```python
from build123d import *

# Parameters (mm, degrees)
F0_W     = 14.2082790844
F0_H     = 68.7680318952
F0_W_2   = 16.8297942728
F1_DEPTH = 25.4
F2_R     = 10.9503541364
F3_DEPTH = 9.4174239784
F5_W     = 35.7930406462
F5_H     = 20.7620039582
F6_DEPTH = 71.0562486202


with BuildPart() as f1:
    # F0 (on Top) → F1 (new body)
    with BuildSketch(Plane.XY):
        Polygon((3.0717435293, 45.1143532991), (19.8212694377, 45.1143532991), (19.8212694377, 99.9910533428), (-35.7833579183, 99.9910533428), (-35.7833579183, 72.552703321), (-11.1365355551, 72.552703321), (-11.1365355551, 45.1143532991), align=None)
        with Locations((-4.0323960129, 10.7303373516)):
            Rectangle(F0_W, F0_H)
        with Locations((-19.5514326915, 10.7303373516)):
            Rectangle(F0_W_2, F0_H)
        Polygon((-27.9663298279, 45.1143532991), (-11.1365355551, 45.1143532991), (-11.1365355551, 72.552703321), (-35.7833579183, 72.552703321), (-35.7833579183, 45.1143532991), align=None)
        Polygon((-27.9663298279, -23.653678596), (-27.9663298279, 45.1143532991), (-35.7833579183, 45.1143532991), (-35.7833579183, 0), (-35.7833579183, -47.0235422254), (-11.1365355551, -47.0235422254), (-11.1365355551, -23.653678596), align=None)
    extrude(amount=F1_DEPTH)

    # F2 (on face) → F3 (join)
    with BuildSketch(Plane.XY.offset(25.4)):
        with Locations((-13.6862043291, 22.343069315)):
            Circle(F2_R)
    extrude(amount=F3_DEPTH)

    # F5 (on face) → F6 (join)
    with BuildSketch(Plane.XY.offset(25.4)):
        with Locations((-6.4500138396, 73.0364732444)):
            Rectangle(F5_W, F5_H)
    extrude(amount=F6_DEPTH)


solid = f1.part
```
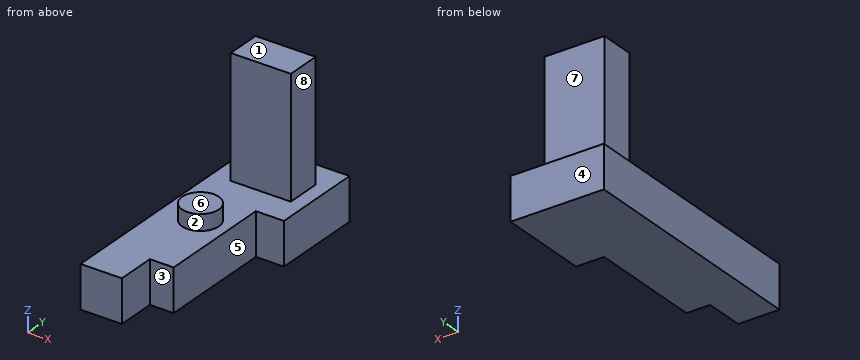
CAD build for the part. Positions are in the model's coordinates, mm. Face numbers are marked on the shaded views. A direction names the side the tool comes from. Give positions to 0.01 mm unless a question says otherwise; leave off trailing zeros. Loops run counter-clockwise (first coordinate to the right, second up) from the corner with the lowest first, then second, coordinate; pieces in that order, holes last. Notation, with made-up numbers: M 55.25,40.25 L 84.25,40.25 A15 cw 84.25,59.25 Z; hole C 56.5,-39.75 d11. An arc over 180 degrees is marked long. Use one line per item in the form item = value.
Item 1: Slice it at D-D (y = 6). List the corners of the cut face in (x, z), plus the area to 3 significant figures.
Determined:
outline = M -35.78,0 L 3.07,0 L 3.07,25.4 L -35.78,25.4 Z
area = 987 mm2
Item 2: Two-plate mould, pull along Y, no slides. Class the marked faces 1, 2, 3 and 4: pulls with the +Y half, pulls with the -Y half, needs draft (parallel to the pull), parting line crosses it, or undercut.
Determined:
face_1 = needs draft
face_2 = undercut
face_3 = pulls with the -Y half
face_4 = pulls with the +Y half
Item 3: Flat gauge pins, fed straight in: pin 1 (12 mm diameter, centred on x = 2.5, z = 44, fed in from +Y); pin 2 (10.5 mm diameter, centred on y = 77.5, z = 71.5, fed in from -X); pin 3 (3 mm diameter, centred on x = -1.5, y = 28.5, fed in from +Z); pin 4 (4 mm diameter, centred on x = 6.5, y = 18.5, fed in from +Z). Where does each tip first touch, or does it go through?
Determined:
pin_1 = 83.42
pin_2 = -24.35
pin_3 = 25.4
pin_4 = through
Item 4: Drill centre lines: probe 1 along Z at (x, y) = (-8, 46); probe 2 along Y at (x, z) = (-1, 35); probe 3 along X at (y, z) = (64.5, 65). Where is each one in solid material? Low to high. Write a range as from..to.
Determined:
probe_1 = 0..25.4
probe_2 = 62.66..83.42
probe_3 = -24.35..11.45
Item 5: Slice it at A-A (z = 28.5). List the corners of the cut face in (x, y), plus the area to 3 significant figures.
Determined:
outline = C -13.69,22.34 d21.9; M -24.35,62.66 L 11.45,62.66 L 11.45,83.42 L -24.35,83.42 Z
area = 1,120 mm2
Item 6: Which spindle directions (+Z, -Z, +X, -X, +Y, -Y) get a long thin tool onto all of the face, cutting with end or side? Do the marked faces 5, 6, 7 and 8. Say none if no direction does.
Determined:
face_5 = +Z, -Z, +X, -Y
face_6 = +Z, +X, -X, -Y
face_7 = +Z, +X, -X, +Y
face_8 = +Z, +X, +Y, -Y
Item 7: Slice it at B-B (x = 9.5). List the corners of the cut face in (y, z), plus the area to 3 significant figures.
Determined:
outline = M 45.11,0 L 99.99,0 L 99.99,25.4 L 83.42,25.4 L 83.42,96.46 L 62.66,96.46 L 62.66,25.4 L 45.11,25.4 Z
area = 2,870 mm2
Item 8: Slice it at C-C (z = 11.5). List the corners of the cut face in (x, y), plus the area to 3 significant figures.
Determined:
outline = M -35.78,-47.02 L -11.14,-47.02 L -11.14,-23.65 L 3.07,-23.65 L 3.07,45.11 L 19.82,45.11 L 19.82,99.99 L -35.78,99.99 Z
area = 6,300 mm2
